```python
from build123d import *

# Parameters (mm, degrees)
F0_R     = 1.5
F0_R_2   = 3.5
F1_DEPTH = 1.5
F2_R     = 3


with BuildPart() as f1:
    # F0 (on Top) → F1 (new body)
    with BuildSketch(Plane.XY):
        with BuildLine():
            ThreePointArc((-13, 62), (-16.535534, 60.535534), (-18, 57))
            Line((-18, 57), (-18, 18.154738))
            ThreePointArc((-18, 18.154738), (-19.25, 15.25), (-18, 12.345262))
            Line((-18, 12.345262), (-18, -12.345262))
            ThreePointArc((-18, -12.345262), (-19.25, -15.25), (-18, -18.154738))
            Line((-18, -18.154738), (-18, -50.25))
            ThreePointArc((-18, -50.25), (-16.535534, -53.785534), (-13, -55.25))
            Line((-13, -55.25), (-10, -55.25))
            Line((-10, -55.25), (-7.663217, -47.453241))
            ThreePointArc((-7.663217, -47.453241), (0, -41.75), (7.663217, -47.453241))
            Line((7.663217, -47.453241), (10, -55.25))
            Line((10, -55.25), (13, -55.25))
            ThreePointArc((13, -55.25), (16.535534, -53.785534), (18, -50.25))
            Line((18, -50.25), (18, -18.154738))
            ThreePointArc((18, -18.154738), (19.25, -15.25), (18, -12.345262))
            Line((18, -12.345262), (18, 12.345262))
            ThreePointArc((18, 12.345262), (19.25, 15.25), (18, 18.154738))
            Line((18, 18.154738), (18, 57))
            ThreePointArc((18, 57), (16.535534, 60.535534), (13, 62))
            Line((13, 62), (10.908712, 62))
            ThreePointArc((10.908712, 62), (8.208403, 62.791873), (6.363415, 64.916667))
            ThreePointArc((6.363415, 64.916667), (0, 69), (-6.363415, 64.916667))
            ThreePointArc((-6.363415, 64.916667), (-8.208403, 62.791873), (-10.908712, 62))
            Line((-10.908712, 62), (-13, 62))
        make_face()
        with Locations((-13, -44.75)):
            Circle(F0_R, mode=Mode.SUBTRACT)
        with Locations((-15.25, -15.25)):
            Circle(F0_R, mode=Mode.SUBTRACT)
        with Locations((13, -44.75)):
            Circle(F0_R, mode=Mode.SUBTRACT)
        with Locations((15.25, -15.25)):
            Circle(F0_R, mode=Mode.SUBTRACT)
        with Locations((-15.25, 15.25)):
            Circle(F0_R, mode=Mode.SUBTRACT)
        with Locations((-13, 57)):
            Circle(F0_R, mode=Mode.SUBTRACT)
        with Locations((15.25, 15.25)):
            Circle(F0_R, mode=Mode.SUBTRACT)
        with Locations((0, 62)):
            Circle(F0_R_2, mode=Mode.SUBTRACT)
        with Locations((13, 57)):
            Circle(F0_R, mode=Mode.SUBTRACT)
    extrude(amount=F1_DEPTH)

    # F2
    f2_edges = [f1.edges().sort_by_distance(p)[0] for p in [
        (-18, 12.345262, 0.75),
        (-18, 18.154738, 0.75),
        (-18, -12.345262, 0.75),
        (-18, -18.154738, 0.75),
        (18, -18.154738, 0.75),
        (18, -12.345262, 0.75),
        (18, 12.345262, 0.75),
        (18, 18.154738, 0.75),
        (-10, -55.25, 0.75),
        (10, -55.25, 0.75),
    ]]
    fillet(f2_edges, radius=F2_R)


solid = f1.part
```
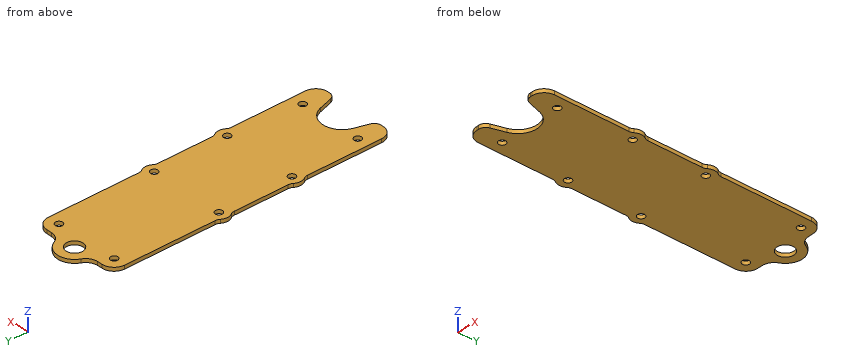
Work out the finished part from the listing and answer in its coordinate system (mm). Round coordinates to 2 decimals unless told otherwise and drop trailing zeros. Write each loop counter-clockwise with the first axis right and the second up, starting at its lowest first coordinate (ties: lowest second). Pieces come first, ordered by that corner, then holes. Notation, with made-up numbers: (5.5, 69) - (43.5, 69) arc R9 ccw to (43.5, 80) - close; hole circle Ø4 at (85.25, 57). An arc over 180 degrees is marked (long way). Return JSON: item names as keys, results as strings. Group by question number.
Q1. This flat-tipped pin is pushed along its axis until it touches: pin 1 Ø0.8 at (y, z) = (-36.5, 0.5) entering from +X. Where does it stop, or does it pass through?
Q2. Find the intervals of material crossed by L1, parallel to Y at x = -13, z = 0.75; L2, parallel to X at y = 15.5, z = 1.4; L3, parallel to Y at x = 0, z = 0.6, in increasing order.
Q3. The part is cut by section A-A on y = -15.25. Write down the section's boundary in (x, z), then the cut area to 4 significant figures.
Q4. The part is cut by section C-C on y = -44.75. Write down the section's boundary in (x, z) (3 decimals).
Q5. The part is cut by section B-B on x = 1. Write down the section's boundary in (y, z).
Q6. The part is cut by section D-D on z = 0.35. Count the separate pieces of the cut face and the enclosed holes in it, then the cut area to 3 significant figures.
Solved:
{
 "1": {"pin 1": "x = 18"},
 "2": {"L1": "-55.25 to -46.25, -43.25 to 55.5, 58.5 to 62", "L2": "-19.24 to -16.73, -13.77 to 13.77, 16.73 to 19.24", "L3": "-41.75 to 58.5, 65.5 to 69"},
 "3": {"outline": "(-19.25, 0) - (-16.75, 0) - (-16.75, 1.5) - (-19.25, 1.5) - close; (-13.75, 0) - (13.75, 0) - (13.75, 1.5) - (-13.75, 1.5) - close; (16.75, 0) - (19.25, 0) - (19.25, 1.5) - (16.75, 1.5) - close", "area": "48.75 mm²"},
 "4": {"outline": "(-18, 0) - (-14.5, 0) - (-14.5, 1.5) - (-18, 1.5) - close; (-11.5, 0) - (-6.245, 0) - (-6.245, 1.5) - (-11.5, 1.5) - close; (6.245, 0) - (11.5, 0) - (11.5, 1.5) - (6.245, 1.5) - close; (14.5, 0) - (18, 0) - (18, 1.5) - (14.5, 1.5) - close"},
 "5": {"outline": "(-41.81, 0) - (58.65, 0) - (58.65, 1.5) - (-41.81, 1.5) - close; (65.35, 0) - (68.93, 0) - (68.93, 1.5) - (65.35, 1.5) - close"},
 "6": {"separate pieces": "1", "enclosed holes": "9", "area": "4,000 mm²"}
}
